Part model, mm, in its own coordinate system. Face numbers are marked on the shaded views. A direction names the side the tool comes from. Give positions to 0.01 mm unless a question says otherwise; leave off trailing zeros. Write each loop counter-clockwise with the first axis right and the second up, starting at its lowest first coordinate (ties: lowest second). Pieces come first, ordered by that corner, then holes.
Solid Edge part; units mm, degrees
sketch "Sketch1" plane through (0, 0, 0) normal (0, -1, 0) x (1, 0, 0)
  line L0 (-253.0269, 43.2231) -> (-3.0269, 43.2231)
  line L1 (-3.0269, 43.2231) -> (-3.0269, 142.8693)
  line L2 (-3.0269, 142.8693) -> (-213.6588, 142.8693)
  line L3 (-355.6424, 426.5914) -> (-213.6588, 142.8693)
  arc A0 (-424.8013, 386.4753) -> (-355.6424, 426.5914) centre (-408.7684, 438.5071) ccw
  line L4 (-303.0701, 143.2231) -> (-424.8013, 386.4753)
  line L5 (-303.0701, 143.2231) -> (-253.0269, 43.2231)
  dimension "D1" = 253.0269
extrude "Protrusion1" add sketch "Sketch1" along normal blind 3
sketch "Sketch2" plane through (-252.7601, 0, 247.3078) normal (0, 1, 0) x (-1, 0, 0)
  line L0 (-199.6901, -204.0847) -> (-149.6901, -204.0847)
  line L1 (-149.6901, -204.0847) -> (-149.6901, -104.0847)
  line L2 (-149.6901, -104.0847) -> (-199.6901, -104.0847)
  line L3 (-199.6901, -104.0847) -> (-199.6901, -204.0847)
extrude "ExtrudedProtrusion_4" add sketch "Sketch2" along normal blind 50
sketch "Sketch3" plane through (-103.0701, 25, 93.223) normal (-1, 0, 0) x (0, -1, 0)
  line L0 (-25, 50) -> (-7.3673, -50)
  line L1 (-7.3673, -50) -> (-25, -50)
  line L2 (-25, -50) -> (-25, 50)
extrude "Cutout1" cut sketch "Sketch3" against normal through all
sketch "Sketch4" plane through (-238.9357, -3, 234.9073) normal (0, -1, 0) x (1, 0, 0)
  arc A0 (-185.8656, 151.5681) -> (-116.7067, 191.6842) centre (-169.8327, 203.5998) ccw
  line L0 (-98.47, 155.2422) -> (-116.7067, 191.6842)
  line L1 (-169.8327, 119.53) -> (-98.47, 155.2422)
  line L2 (-185.8656, 151.5681) -> (-169.8327, 119.53)
extrude "ExtrudedProtrusion_5" add sketch "Sketch4" along normal blind 20
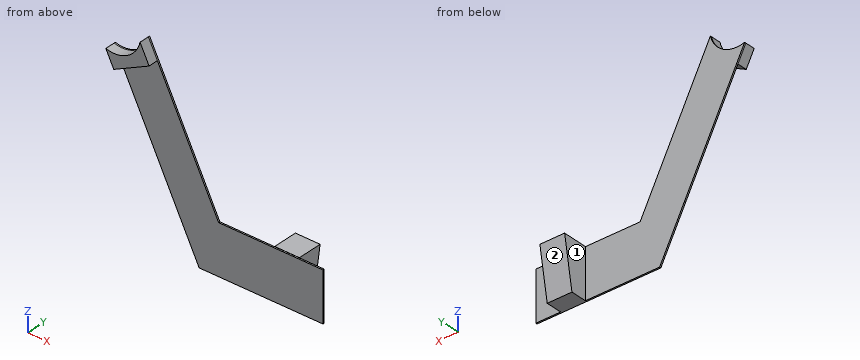
1) 3-axis set-ups, long thin cutter, end or side, ignore diameter. For the marked faces 1 and 2: which of +Z, -Z, +X, -X, +Y, -Y reach the whole face in a straight line?
Check result:
face 1: +Z, -Z, -X, +Y
face 2: -Z, +X, -X, +Y
2) Saw through at D-D (x = -183). Write the cut outline in (y, z).
Check result:
outline: (-3, 43.22) - (0, 43.22) - (0, 142.87) - (-3, 142.87) - close
3) Flat gauge pins, fed straight in: P1, Ø4, axis at x = -185, z = 93.5, coming from the +Y side; P2, Ø15, axis at y = 32, z = 71.5, coming from the -X side; P3, Ø3.5, axis at x = -157, y = -1, coming from the +Z side; P4, Ø10, axis at x = -241.5, z = 217.5, coming from the -Y side. Where does each tip first touch, or does it go through?
Check result:
P1: stops at y = 0
P2: stops at x = -103.07
P3: stops at z = 142.87
P4: passes through
4) Saw through at B-B (y = 15.5). Write the cut outline in (x, z).
Check result:
outline: (-103.07, 43.22) - (-53.07, 43.22) - (-53.07, 143.22) - (-103.07, 143.22) - close
5) Drill centre lines: L1, parallel to Y at x = -358.5, z = 372; L2, parallel to X at y = 0.5, z = 78; L3, parallel to Z at x = -128.5, y = -1.5. Where is each one in solid material? Low to high.
Check result:
L1: y = -3 to 0
L2: x = -103.07 to -53.07
L3: z = 43.22 to 142.87
